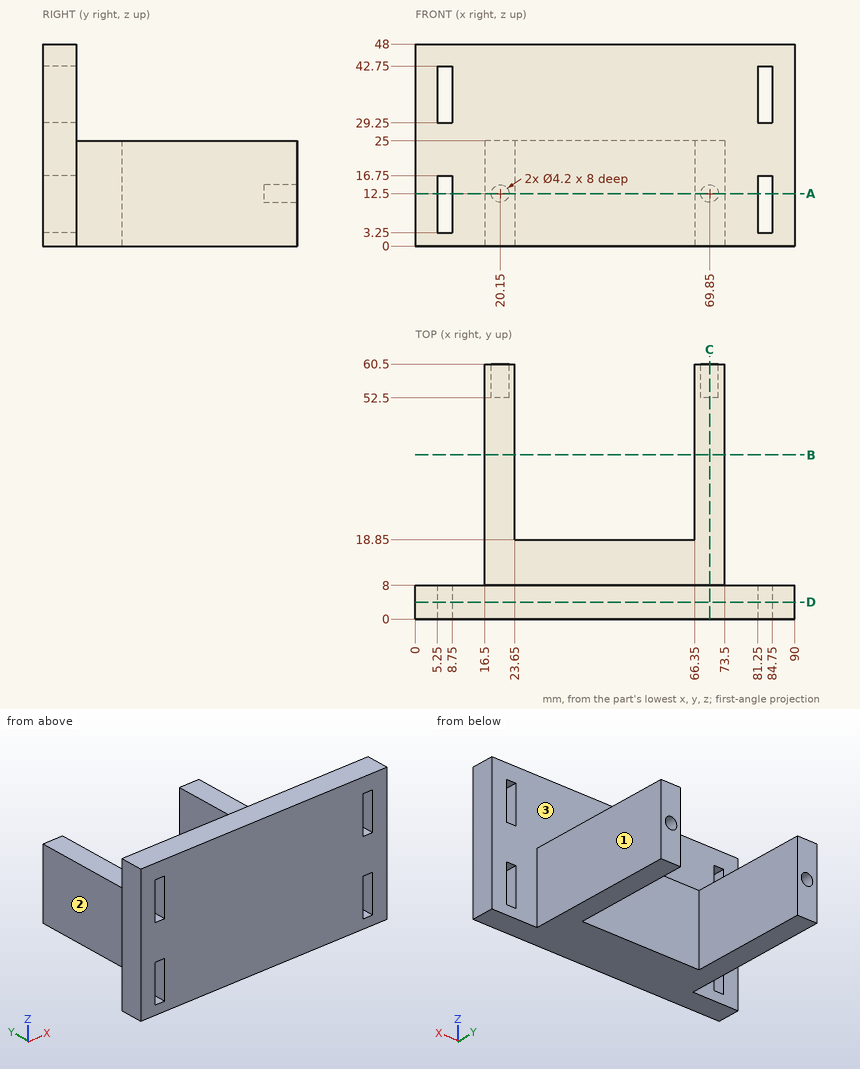
Here's the drawing with two shaded views (mm, measured from the low corner). I have some questions. A direction names the side the tool comes from. Give positions to 0.01 mm unless a question says otherwise; leave off trailing zeros. Loops run counter-clockwise (first coordinate to the right, second up) from the corner with the lowest first, then second, coordinate; pieces in that order, holes last. Notation, with made-up numbers: M 23.5,21 L 55.5,21 A22 cw 55.5,60 Z; hole C 89.25,7 d9. An arc over 180 degrees is marked long. Use one line per item in the form item = value. Start each with the question number.
(1) I want a section at D-D, the plane y = 4. Write out the boundary of the cut face in (x, z).
(2) I want a section at C-C, the plane x = 69.85. Write out the boundary of the cut face in (y, z).
(3) I'm going to push flat-ended pins straight in: P1, Ø3, axis at x = 57.5, y = 17, coming from the +Z side; P2, Ø7.5, axis at x = 49, z = 12.5, coming from the +Y side; P3, Ø3, axis at y = 53, z = 9.5, coming from the -X side; P4, Ø12, axis at x = 41, y = 25.5, coming from the +Z side. Where does each tip first touch, or does it pass through?
(4) On a 3-axis mill with a long thin cutter (end or side, diameter ignored), from which of +Z, -Z, +X, -X, +Y, -Y can I reach the whole of each face in a straight line? I mean the marked faces 1, 2 and 3. Say none if no direction works.
(5) I want a section at B-B, the plane y = 39. Write out the boundary of the cut face in (x, z), and give its area (4 significant figures).
(6) Please list where these lines run through material, in increasing order: line 1 (X direction, y = 56, z = 12.5); line 2 (Z direction, x = 20, y = 56); line 3 (X direction, y = 40.5, z = 16).
(7) I want a section at A-A, the plane z = 12.5. Write out the boundary of the cut face in (x, y), and give its area (3 significant figures).
Worked out:
q1.outline = M 0,0 L 90,0 L 90,48 L 0,48 Z; hole M 5.25,3.25 L 8.75,3.25 L 8.75,16.75 L 5.25,16.75 Z; hole M 5.25,29.25 L 8.75,29.25 L 8.75,42.75 L 5.25,42.75 Z; hole M 81.25,3.25 L 84.75,3.25 L 84.75,16.75 L 81.25,16.75 Z; hole M 81.25,29.25 L 84.75,29.25 L 84.75,42.75 L 81.25,42.75 Z
q2.outline = M 0,0 L 60.5,0 L 60.5,10.4 L 52.5,10.4 L 52.5,14.6 L 60.5,14.6 L 60.5,25 L 8,25 L 8,48 L 0,48 Z
q3.P1 = 25
q3.P2 = 18.85
q3.P3 = 16.5
q3.P4 = through
q4.face_1 = +Z, -Z, +X, +Y
q4.face_2 = +Z, -Z, -X, +Y
q4.face_3 = +Z, +Y
q5.outline = M 16.5,0 L 23.65,0 L 23.65,25 L 16.5,25 Z; M 66.35,0 L 73.5,0 L 73.5,25 L 66.35,25 Z
q5.area = 357.5 mm²
q6.line_1 = 16.5 to 18.05, 22.25 to 23.65, 66.35 to 67.75, 71.95 to 73.5
q6.line_2 = 0 to 10.41, 14.59 to 25
q6.line_3 = 16.5 to 23.65, 66.35 to 73.5
q7.outline = M 0,0 L 5.25,0 L 5.25,8 L 0,8 Z; M 8.75,0 L 81.25,0 L 81.25,8 L 73.5,8 L 73.5,60.5 L 71.95,60.5 L 71.95,52.5 L 67.75,52.5 L 67.75,60.5 L 66.35,60.5 L 66.35,18.85 L 23.65,18.85 L 23.65,60.5 L 22.25,60.5 L 22.25,52.5 L 18.05,52.5 L 18.05,60.5 L 16.5,60.5 L 16.5,8 L 8.75,8 Z; M 84.75,0 L 90,0 L 90,8 L 84.75,8 Z
q7.area = 1,810 mm²
